The listing builds one solid part. Answer for the finished solid, in the listing's coordinates (mm). A direction names the side the tool comes from. Round coordinates to 2 decimals unless told otherwise and drop trailing zeros. Loops run counter-clockwise (first coordinate to the right, second up) from the corner with the lowest first, then second, coordinate; pieces in that order, holes last. Notation, with made-up numbers: M 34.5,1.25 L 80.5,1.25 A12 cw 80.5,18.25 Z; hole C 58,-32 d4. An arc over 180 degrees is marked long. Answer as a JSON object with one key per item and string values.
```python
from build123d import *

# Parameters (mm, degrees)
F2_R     = 25.4
F3_R     = 25.4
F3_R_2   = 3.175
F4_DEPTH = 82.551


with BuildPart() as f1:
    # F0 (on Top) → F1 (revolve)
    with BuildSketch(Plane.XY):
        Polygon((0, 3.175), (0, 0), (0, -3.175), (76.2, -3.175), (82.866636, -79.375), (139.7, -79.375), (139.7, 0), (139.7, 79.375), (82.866636, 79.375), (76.2, 3.175), align=None)
    revolve(axis=Axis((0, 1.5875, 0), (0, 1, 0)))

    # F2
    f2_edges = [f1.edges().sort_by_distance(p)[0] for p in [
        (-139.7, -79.375, 0),
        (-139.7, 79.375, 0),
    ]]
    fillet(f2_edges, radius=F2_R)

    # F3 (on face) → F4 (cut, through all)
    with BuildSketch(Plane.XZ.offset(3.175)):
        Circle(F3_R)
        with Locations((0, 31.75)):
            Circle(F3_R_2)
        with Locations((-27.496307, -15.875)):
            Circle(F3_R_2)
        with Locations((27.496307, -15.875)):
            Circle(F3_R_2)
    extrude(amount=-F4_DEPTH, mode=Mode.SUBTRACT)


solid = f1.part
```
Item 1: Straight lines are drawn through the part: line 1 (Z direction, x = 0, y = 0) (3 decimals); line 2 (Y direction, x = 0.5, z = -51) (3 decimals); line 3 (Z direction, x = 42, y = -24). For each, find the intervals that lie inside material, in ascending order.
Values follow:
{"line 1": "-139.7 to -25.4, 25.4 to 28.575, 34.925 to 139.7", "line 2": "-3.175 to 3.175", "line 3": "-133.24 to -65.75, 65.75 to 133.24"}
Item 2: The part is cut by section C-C (y = -36). Give the vertices of the cut face in (x, z), then the cut area to 3 significant figures.
Values follow:
{"outline": "C 0,0 d279.4; hole C 0,0 d158.14", "area": "41,700 mm^2"}
Item 3: Which of the six approach directions +Z, -Z, +X, -X, +Y, -Y give full straight-line access (tool end or side, diameter ignored) to faces 1 (the face through (76, 79.375, -34)), 2 (the face through (-33, -3.175, -1)), 3 (the face through (33, 3.175, -1))?
Values follow:
{"face 1": "+Z, -Z, +X, -X, +Y", "face 2": "-Y", "face 3": "+Y"}
Item 4: Determine the mould class of faces 4 (the face through (-5.506, -0.044, -24.796)), 5 (the face through (-76, -79.375, -34)), 6 (the face through (-110.86, 0.76, 85.01)) for opening direction X: released by +X, released by -X, zero draft, split by the parting line, or undercut.
Values follow:
{"face 4": "undercut", "face 5": "zero draft", "face 6": "split by the parting line"}
Item 5: Flat-ended cylindrical pins translate along their axes: P1, Ø12, axis at x = -17, z = 52, coming from the -Y side (3 decimals); P2, Ø8.5, axis at x = 27.5, z = -15.88, coming from the +Y side (3 decimals); P3, Ø10, axis at y = 3.5, z = -93.5, coming from the +X side. Find the tip coordinate at first contact, or state that the pin passes through.
Values follow:
{"P1": "y = -3.175", "P2": "y = 3.175", "P3": "x = 108.09"}
Item 6: The part is cut by section B-B (y = 34.5). Give the vertices of the cut face in (x, z), then the cut area to 3 significant figures.
Values follow:
{"outline": "C 0,0 d279.4; hole C 0,0 d157.88", "area": "41,700 mm^2"}
Item 7: The part is cut by section A-A (z = 0). Give the vertices of the cut face in (x, y) (3 decimals), then the cut area to 3 significant figures.
Values follow:
{"outline": "M -139.7,-53.975 A25.4 ccw -114.3,-79.375 L -82.867,-79.375 L -76.2,-3.175 L -25.4,-3.175 L -25.4,3.175 L -76.2,3.175 L -82.867,79.375 L -114.3,79.375 A25.4 ccw -139.7,53.975 Z; M 25.4,-3.175 L 76.2,-3.175 L 82.867,-79.375 L 114.3,-79.375 A25.4 ccw 139.7,-53.975 L 139.7,53.975 A25.4 ccw 114.3,79.375 L 82.867,79.375 L 76.2,3.175 L 25.4,3.175 Z", "area": "19,200 mm^2"}
